from build123d import *

# Parameters (mm, degrees)
F0_R     = 50
F1_DEPTH = 30
F2_DEPTH = 10


with BuildPart() as f1:
    # F0 (on Front) → F1 (new body)
    with BuildSketch(Plane.XZ):
        Circle(F0_R)
        with BuildLine():
            ThreePointArc((28.5316954889, 9.2705098312), (29.6306502179, 4.6930339512), (30, 0))
            ThreePointArc((30, 0), (29.6306502179, -4.6930339512), (28.5316954889, -9.2705098312))
            ThreePointArc((28.5316954889, -9.2705098312), (24.2705098312, -17.6335575688), (17.6335575688, -24.2705098312))
            ThreePointArc((17.6335575688, -24.2705098312), (9.2705098312, -28.5316954889), (0, -30))
            ThreePointArc((0, -30), (-9.2705098312, -28.5316954889), (-17.6335575688, -24.2705098312))
            ThreePointArc((-17.6335575688, -24.2705098312), (-24.2705098312, -17.6335575688), (-28.5316954889, -9.2705098312))
            ThreePointArc((-28.5316954889, -9.2705098312), (-30, 0), (-28.5316954889, 9.2705098312))
            ThreePointArc((-28.5316954889, 9.2705098312), (-24.2705098312, 17.6335575688), (-17.6335575688, 24.2705098312))
            ThreePointArc((-17.6335575688, 24.2705098312), (-9.2705098312, 28.5316954889), (0, 30))
            ThreePointArc((0, 30), (9.2705098312, 28.5316954889), (17.6335575688, 24.2705098312))
            ThreePointArc((17.6335575688, 24.2705098312), (24.2705098312, 17.6335575688), (28.5316954889, 9.2705098312))
        make_face(mode=Mode.SUBTRACT)
    extrude(amount=F1_DEPTH)

    # F0 (on Front) → F2 (join)
    with BuildSketch(Plane.XZ):
        with BuildLine():
            Line((-7.6705975424, 10.5576717766), (-17.6335575688, 24.2705098312))
            ThreePointArc((-17.6335575688, 24.2705098312), (-24.2705098312, 17.6335575688), (-28.5316954889, 9.2705098312))
            Line((-28.5316954889, 9.2705098312), (-12.4112875377, 4.0326717766))
            ThreePointArc((-12.4112875377, 4.0326717766), (-10.5576717766, 7.6705975424), (-7.6705975424, 10.5576717766))
        make_face()
        with BuildLine():
            Line((-4.731671281, 6.5125868047), (-7.6705975424, 10.5576717766))
            ThreePointArc((-7.6705975424, 10.5576717766), (-10.5576717766, 7.6705975424), (-12.4112875377, 4.0326717766))
            Line((-12.4112875377, 4.0326717766), (-7.6560049562, 2.4875868047))
            ThreePointArc((-7.6560049562, 2.4875868047), (-6.5125868047, 4.731671281), (-4.731671281, 6.5125868047))
        make_face()
        with BuildLine():
            Line((0, 8.05), (0, 13.05))
            ThreePointArc((0, 13.05), (-4.0326717766, 12.4112875377), (-7.6705975424, 10.5576717766))
            Line((-7.6705975424, 10.5576717766), (-4.731671281, 6.5125868047))
            ThreePointArc((-4.731671281, 6.5125868047), (-2.4875868047, 7.6560049562), (0, 8.05))
        make_face()
        with BuildLine():
            Line((4.731671281, 6.5125868047), (7.6705975424, 10.5576717766))
            ThreePointArc((7.6705975424, 10.5576717766), (4.0326717766, 12.4112875377), (0, 13.05))
            Line((0, 13.05), (0, 8.05))
            ThreePointArc((0, 8.05), (2.4875868047, 7.6560049562), (4.731671281, 6.5125868047))
        make_face()
        with BuildLine():
            Line((7.6560049562, 2.4875868047), (12.4112875377, 4.0326717766))
            ThreePointArc((12.4112875377, 4.0326717766), (10.5576717766, 7.6705975424), (7.6705975424, 10.5576717766))
            Line((7.6705975424, 10.5576717766), (4.731671281, 6.5125868047))
            ThreePointArc((4.731671281, 6.5125868047), (6.5125868047, 4.731671281), (7.6560049562, 2.4875868047))
        make_face()
        with BuildLine():
            ThreePointArc((13.05, 0), (12.8893328448, 2.0414697688), (12.4112875377, 4.0326717766))
            Line((12.4112875377, 4.0326717766), (7.6560049562, 2.4875868047))
            ThreePointArc((7.6560049562, 2.4875868047), (7.9508911418, 1.2592974436), (8.05, 0))
            ThreePointArc((8.05, 0), (7.9508911418, -1.2592974436), (7.6560049562, -2.4875868047))
            Line((7.6560049562, -2.4875868047), (12.4112875377, -4.0326717766))
            ThreePointArc((12.4112875377, -4.0326717766), (12.8893328448, -2.0414697688), (13.05, 0))
        make_face()
        with BuildLine():
            ThreePointArc((7.6705975424, -10.5576717766), (10.5576717766, -7.6705975424), (12.4112875377, -4.0326717766))
            Line((12.4112875377, -4.0326717766), (7.6560049562, -2.4875868047))
            ThreePointArc((7.6560049562, -2.4875868047), (6.5125868047, -4.731671281), (4.731671281, -6.5125868047))
            Line((4.731671281, -6.5125868047), (7.6705975424, -10.5576717766))
        make_face()
        with BuildLine():
            ThreePointArc((0, -13.05), (4.0326717766, -12.4112875377), (7.6705975424, -10.5576717766))
            Line((7.6705975424, -10.5576717766), (4.731671281, -6.5125868047))
            ThreePointArc((4.731671281, -6.5125868047), (2.4875868047, -7.6560049562), (0, -8.05))
            Line((0, -8.05), (0, -13.05))
        make_face()
        with BuildLine():
            ThreePointArc((-7.6705975424, -10.5576717766), (-4.0326717766, -12.4112875377), (0, -13.05))
            Line((0, -13.05), (0, -8.05))
            ThreePointArc((0, -8.05), (-2.4875868047, -7.6560049562), (-4.731671281, -6.5125868047))
            Line((-4.731671281, -6.5125868047), (-7.6705975424, -10.5576717766))
        make_face()
        with BuildLine():
            ThreePointArc((-12.4112875377, -4.0326717766), (-10.5576717766, -7.6705975424), (-7.6705975424, -10.5576717766))
            Line((-7.6705975424, -10.5576717766), (-4.731671281, -6.5125868047))
            ThreePointArc((-4.731671281, -6.5125868047), (-6.5125868047, -4.731671281), (-7.6560049562, -2.4875868047))
            Line((-7.6560049562, -2.4875868047), (-12.4112875377, -4.0326717766))
        make_face()
        with BuildLine():
            Line((-7.6560049562, 2.4875868047), (-12.4112875377, 4.0326717766))
            ThreePointArc((-12.4112875377, 4.0326717766), (-13.05, 0), (-12.4112875377, -4.0326717766))
            Line((-12.4112875377, -4.0326717766), (-7.6560049562, -2.4875868047))
            ThreePointArc((-7.6560049562, -2.4875868047), (-8.05, 0), (-7.6560049562, 2.4875868047))
        make_face()
        with BuildLine():
            ThreePointArc((-28.5316954889, -9.2705098312), (-24.2705098312, -17.6335575688), (-17.6335575688, -24.2705098312))
            Line((-17.6335575688, -24.2705098312), (-7.6705975424, -10.5576717766))
            ThreePointArc((-7.6705975424, -10.5576717766), (-10.5576717766, -7.6705975424), (-12.4112875377, -4.0326717766))
            Line((-12.4112875377, -4.0326717766), (-28.5316954889, -9.2705098312))
        make_face()
        with BuildLine():
            ThreePointArc((0, -30), (9.2705098312, -28.5316954889), (17.6335575688, -24.2705098312))
            Line((17.6335575688, -24.2705098312), (7.6705975424, -10.5576717766))
            ThreePointArc((7.6705975424, -10.5576717766), (4.0326717766, -12.4112875377), (0, -13.05))
            Line((0, -13.05), (0, -30))
        make_face()
        with BuildLine():
            ThreePointArc((28.5316954889, -9.2705098312), (29.6306502179, -4.6930339512), (30, 0))
            ThreePointArc((30, 0), (29.6306502179, 4.6930339512), (28.5316954889, 9.2705098312))
            Line((28.5316954889, 9.2705098312), (12.4112875377, 4.0326717766))
            ThreePointArc((12.4112875377, 4.0326717766), (12.8893328448, 2.0414697688), (13.05, 0))
            ThreePointArc((13.05, 0), (12.8893328448, -2.0414697688), (12.4112875377, -4.0326717766))
            Line((12.4112875377, -4.0326717766), (28.5316954889, -9.2705098312))
        make_face()
        with BuildLine():
            Line((7.6705975424, 10.5576717766), (17.6335575688, 24.2705098312))
            ThreePointArc((17.6335575688, 24.2705098312), (9.2705098312, 28.5316954889), (0, 30))
            Line((0, 30), (0, 13.05))
            ThreePointArc((0, 13.05), (4.0326717766, 12.4112875377), (7.6705975424, 10.5576717766))
        make_face()
    extrude(amount=F2_DEPTH)


solid = f1.part
Could you check a few things on this model? Use its own coordinates, in mm. A direction names the side the tool comes from. Give positions to 0.01 mm unless a question says otherwise; leave off trailing zeros. Order: outer loops, then holes, each group sorted by start corner. A loop starts at its lowest first (then second) coordinate and runs counter-clockwise, first axis right, second up. Notation, with made-up numbers: (58, -39.75) - (72, -39.75) arc R22 cw to (72, -17.75) - close; hole circle Ø9 at (-14, -2.75). An arc over 180 degrees is marked (long way). Return JSON: item names as keys, results as strings. Group by question number.
Q1. Which directions (+Z, -Z, +X, -X, +Y, -Y) give clear straight access to the entire face, cutting with the end or side of a thin tool? Please do faces 1 (the face through (-6, -10, -6)), 2 (the face through (-1, 0, -10)), 3 (the face through (0, -5, 22)).
Q2. Suppose I cut it at A-A, the plane y = -21. Please give me the cut outline in (x, z).
Q3. Thinking about a two-plate mould opening in X: for faces 4 (the face through (47.69, -14.79, 15.02)), 5 (the face through (22, -30, -22)), 6 (the face through (20.584, -4.93, 6.688)), 7 (the face through (20.359, -4.93, -6.615)), which applies, pulls with the +X half, pulls with the -X half, needs draft (parallel to the pull), parting line crosses it, or undercut?
Q4. Suppose I cut it at B-B, the plane y = -6. Please give me the cut outline in (x, z), and give its area (3 significant figures).
Q5. Please list where these lines run through material, in increasing order: line 1 along Z through (x, y) = (0, -10.75); line 2 along Y through (x, z) = (-17.5, -13); line 3 along X through (y, z) = (-14, 2). Write a range as [from, to].
Q6. Will these pins go through, and if not, where does the flat tip stop? pin 1 Ø17.5 at (x, z) = (4.5, 2.5) entering from -Y; pin 2 Ø4 at (x, y) = (36.5, -17.5) entering from +Z; pin 3 Ø11 at (y, z) = (-4, -17.5) entering from -X.
Q7. Suppose I cut it at C-C, the plane z = -27. Please give me the cut outline in (x, y), and give its area (3 significant figures).
Q8. Suppose I cut it at D-D, the plane x = 14. Please give me the cut outline in (y, z), and give its area (3 significant figures).
Resolved:
{
 "1": {"face 1": "-Y", "face 2": "+Z, -Z, +X, -X, +Y", "face 3": "+Y, -Y"},
 "2": {"outline": "circle Ø100 at (0, 0); hole circle Ø60 at (0, 0)"},
 "3": {"face 4": "parting line crosses it", "face 5": "needs draft", "face 6": "undercut", "face 7": "undercut"},
 "4": {"outline": "circle Ø100 at (0, 0); hole (-28.53, -9.27) - (-12.41, -4.03) arc R13.05 cw to (-12.41, 4.03) - (-28.53, 9.27) arc R30 ccw to start; hole (-17.63, -24.27) arc R30 ccw to (0, -30) - (0, -13.05) arc R13.05 cw to (-7.67, -10.56) - close; hole (-17.63, 24.27) - (-7.67, 10.56) arc R13.05 cw to (0, 13.05) - (0, 30) arc R30 ccw to start; hole circle Ø16.1 at (0, 0); hole (7.67, -10.56) - (17.63, -24.27) arc R30 ccw to (28.53, -9.27) - (12.41, -4.03) arc R13.05 cw to start; hole (7.67, 10.56) arc R13.05 cw to (12.41, 4.03) - (28.53, 9.27) arc R30 ccw to (17.63, 24.27) - close", "area": "6,500 mm2"},
 "5": {"line 1": "z = [-50, -30], [30, 50]", "line 2": "y = [-10, 0]", "line 3": "x = [-49.96, -29.93], [29.93, 49.96]"},
 "6": {"pin 1": "stops at y = -10", "pin 2": "stops at z = 36.19", "pin 3": "stops at x = -48.54"},
 "7": {"outline": "(-42.08, -30) - (-13.08, -30) - (-13.08, 0) - (-42.08, 0) - close; (0, -10) - (13.08, -10) - (13.08, -30) - (42.08, -30) - (42.08, 0) - (0, 0) - close", "area": "1,870 mm2"},
 "8": {"outline": "(-30, -48) - (0, -48) - (0, -19.27) - (-10, -19.27) - (-10, -26.53) - (-30, -26.53) - close; (-30, 26.53) - (-10, 26.53) - (-10, 19.27) - (0, 19.27) - (0, 48) - (-30, 48) - close; (-10, -4.55) - (0, -4.55) - (0, 4.55) - (-10, 4.55) - close", "area": "1,520 mm2"}
}
